Work out the finished part from the listing and answer in its coordinate system (mm). Round coordinates to 2 decimals unless told otherwise and drop trailing zeros. Loops run counter-clockwise (first coordinate to the right, second up) from the corner with the lowest first, then second, coordinate; pieces in that order, holes last. Notation, with made-up numbers: (32.25, -28) -> (59.25, -28) arc R11 ccw to (59.25, -19) -> close; hole circle Ø4 at (19, 47.25). An arc over 180 degrees is marked (long way). Write item = value, one per line. Start each with the question number.
```python
from build123d import *

# Parameters (mm, degrees)
MODEL_R             = 14.2621
BOSS_EXTRUDE1_DEPTH = 5.08


with BuildPart() as part:
    # Model → Boss-Extrude1 (new body)
    with BuildSketch(Plane.XY):
        with BuildLine():
            Line((293.6621, 222.25), (293.6621, 31.75))
            ThreePointArc((293.6621, 31.75), (284.54358689, 11.537102056), (263.355763082, 4.996104661))
            Line((263.355763082, 4.996104661), (212.555763082, 11.346104661))
            ThreePointArc((212.555763082, 11.346104661), (206.870950218, 12.694664017), (201.61011558, 15.236184928))
            Line((201.61011558, 15.236184928), (155.853864238, 43.833842015))
            Line((155.853864238, 43.833842015), (60.155763082, 55.796104661))
            ThreePointArc((60.155763082, 55.796104661), (36.746104661, 85.894236918), (66.844236918, 109.303895339))
            Line((66.844236918, 109.303895339), (168.444236918, 96.603895339))
            ThreePointArc((168.444236918, 96.603895339), (174.129049782, 95.255335983), (179.38988442, 92.713815072))
            Line((179.38988442, 92.713815072), (225.146135762, 64.116157985))
            Line((225.146135762, 64.116157985), (239.7379, 62.292187455))
            Line((239.7379, 62.292187455), (239.7379, 222.25))
            ThreePointArc((239.7379, 222.25), (266.7, 249.2121), (293.6621, 222.25))
        make_face()
        with Locations((63.5, 82.55)):
            Circle(MODEL_R, mode=Mode.SUBTRACT)
        with Locations((114.3, 76.2)):
            Circle(MODEL_R, mode=Mode.SUBTRACT)
        with Locations((165.1, 69.85)):
            Circle(MODEL_R, mode=Mode.SUBTRACT)
        with Locations((215.9, 38.1)):
            Circle(MODEL_R, mode=Mode.SUBTRACT)
        with Locations((266.7, 222.25)):
            Circle(MODEL_R, mode=Mode.SUBTRACT)
        with Locations((266.7, 31.75)):
            Circle(MODEL_R, mode=Mode.SUBTRACT)
    extrude(amount=BOSS_EXTRUDE1_DEPTH)


solid = part.part
```
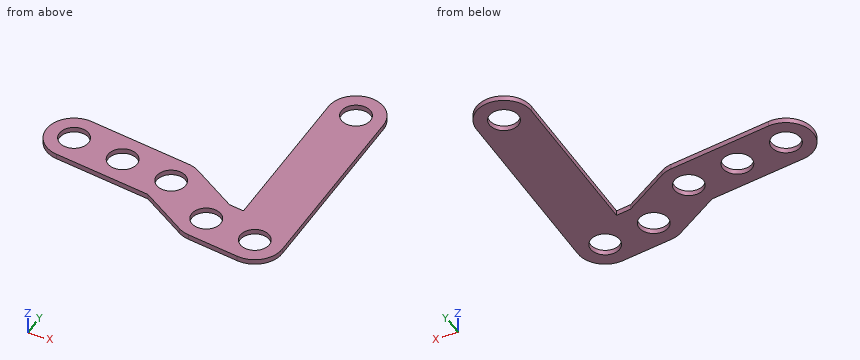
Item 1: Find the intervals of material crossed by line 1 along Y through (x, z) = (266.7, 3.5); line 2 along X through (y, z) = (223.5, 1.8); line 3 along X through (y, z) = (64.5, 3.75), in increasing order. Write a range as [from, to].
Item 2: Section C-C (x = 165.1) is taken. Determine the outline of the cut face in (y, z) (3 decimals).
Item 3: Section A-A (x = 266.7) is taken. Determine the outline of the cut face in (y, z).
Item 4: Flat-ended cylindrical pins translate along their axes: pin 1 (1.5 mm diameter, centred on y = 105, z = 2, fed in from -X); pin 2 (1 mm diameter, centred on y = 74.5, z = 3.5, fed in from -X); pin 3 (2 mm diameter, centred on x = 234, z = 1, fed in from -Y). Find the tip coordinate at first contact, or state that the pin passes through.
Item 5: Section D-D (y = 38.1) is taken. Determine the outline of the cut face in (x, z).
Item 6: Section B-B (z = 2.75) is taken. Determine the outline of the cut face in (x, y), then the cut area to 3 significant figures.
Worked answers:
q1.line_1 = [4.79, 17.49], [46.01, 207.99], [236.51, 249.21]
q1.line_2 = [239.77, 252.49], [280.91, 293.63]
q1.line_3 = [43.47, 106.14], [122.46, 151.88], [178.32, 224.53], [239.74, 293.66]
q2.outline = (38.055, 0) -> (55.588, 0) -> (55.588, 5.08) -> (38.055, 5.08) -> close; (84.112, 0) -> (97.022, 0) -> (97.022, 5.08) -> (84.112, 5.08) -> close
q3.outline = (4.79, 0) -> (17.49, 0) -> (17.49, 5.08) -> (4.79, 5.08) -> close; (46.01, 0) -> (207.99, 0) -> (207.99, 5.08) -> (46.01, 5.08) -> close; (236.51, 0) -> (249.21, 0) -> (249.21, 5.08) -> (236.51, 5.08) -> close
q4.pin_1 = 47.5
q4.pin_2 = 37.62
q4.pin_3 = 8.54
q5.outline = (165.03, 0) -> (201.64, 0) -> (201.64, 5.08) -> (165.03, 5.08) -> close; (230.16, 0) -> (253.93, 0) -> (253.93, 5.08) -> (230.16, 5.08) -> close; (279.47, 0) -> (293.66, 0) -> (293.66, 5.08) -> (279.47, 5.08) -> close
q6.outline = (60.16, 55.8) -> (155.85, 43.83) -> (201.61, 15.24) arc R26.96 ccw to (212.56, 11.35) -> (263.36, 5) arc R26.96 ccw to (293.66, 31.75) -> (293.66, 222.25) arc R26.96 ccw to (239.74, 222.25) -> (239.74, 62.29) -> (225.15, 64.12) -> (179.39, 92.71) arc R26.96 ccw to (168.44, 96.6) -> (66.84, 109.3) arc R26.96 ccw to start; hole circle Ø28.52 at (63.5, 82.55); hole circle Ø28.52 at (114.3, 76.2); hole circle Ø28.52 at (165.1, 69.85); hole circle Ø28.52 at (215.9, 38.1); hole circle Ø28.52 at (266.7, 31.75); hole circle Ø28.52 at (266.7, 222.25)
q6.area = 20,000 mm2
